Answer from the drawing. Dimensions are ordinates in mm from the lowest x, y and z of the part. A direction names the side the tool comes from. Coordinates: 2 decimals unless noted, no trailing zeros. Write each loop counter-clockwise with the first axis right and the second up, starting at its lowest first coordinate (ties: lowest second). Pieces come first, ordered by that corner, then holes. Notation, with made-up numbers: (51.5, 25) - (56.5, 25) arc R20 cw to (56.5, 61) - close; hole circle Ø1 at (-18, 24). An arc over 180 degrees is marked (long way). Use one line per item in the form item = value. Start each with the question number.
Item 1: Given pin 1 (6 mm diameter, centred on y = 6, z = 10.5, fed in from +X); pin 2 (1.5 mm diameter, centred on y = 10.5, z = 75, fed in from -X); pin 3 (5 mm diameter, centred on y = 35, z = 70.5, fed in from +X), each flat-ended and moving along its own axis, determine where each tip first touches the part or whether it passes through.
Item 2: A cutting plane is placed at D-D (y = 8). Write down the section's boundary in (x, z).
Item 3: Determine the mould class of the marked faces 3, 4 and 5 for opening direction X: released by +X, released by -X, zero draft, split by the parting line, or undercut.
Item 4: A cutting plane is placed at A-A (x = 25.4). Write down the section's boundary in (y, z) (3 decimals).
Item 5: A cutting plane is placed at C-C (z = 64). Write down the section's boundary in (x, y) (3 decimals).
Item 6: For the marked faces 1 and 2, determine the directions among +Z, -Z, +X, -X, +Y, -Y from which every point of the face is accessible in a straight line to the end or side of a thin tool.
Item 7: Consider probe 1 along Y at (x, z) = (25, 29); probe 2 along X at (y, z) = (28, 35.5); probe 3 along Z at (x, y) = (34, 7.5). Determine where each line is inside the solid, lowest interval first.
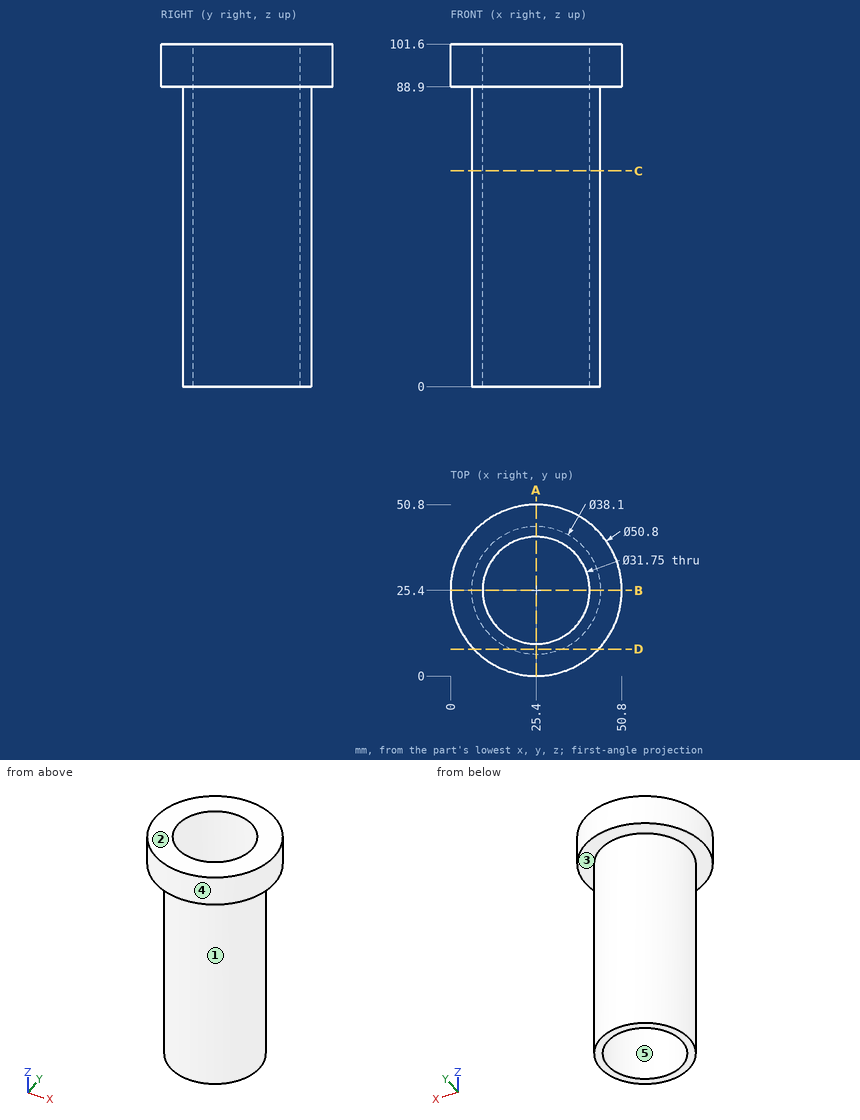
Answer:
q1.pin_1 = 35.09
q1.pin_2 = 12.65
q1.pin_3 = 43.08
q2.outline = (6.9, 88.9) - (17.64, 88.9) - (17.64, 0) - (33.16, 0) - (33.16, 88.9) - (43.9, 88.9) - (43.9, 101.6) - (6.9, 101.6) - close
q3.face_3 = zero draft
q3.face_4 = split by the parting line
q3.face_5 = undercut
q4.outline = (0, 88.9) - (6.35, 88.9) - (6.35, 0) - (9.525, 0) - (9.525, 101.6) - (0, 101.6) - close; (41.275, 0) - (44.45, 0) - (44.45, 88.9) - (50.8, 88.9) - (50.8, 101.6) - (41.275, 101.6) - close
q5.outline = circle Ø38.1 at (25.4, 25.4); hole circle Ø31.75 at (25.4, 25.4)
q6.face_1 = -Z
q6.face_2 = +Z, +X, -X, +Y, -Y
q7.probe_1 = 6.35 to 9.53, 41.27 to 44.45
q7.probe_2 = 6.53 to 9.74, 41.06 to 44.27
q7.probe_3 = 88.9 to 101.6
